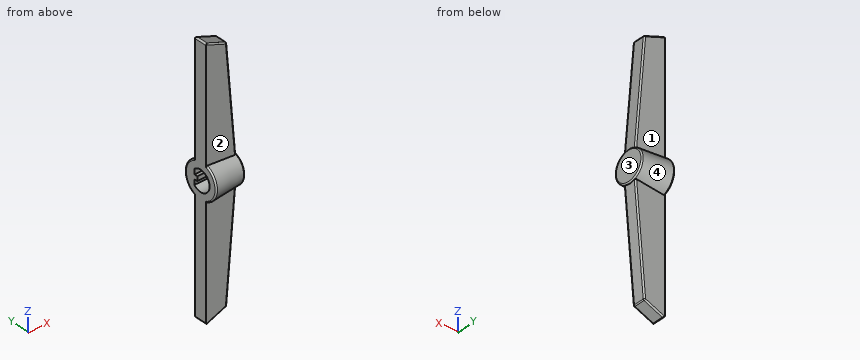
```python
from build123d import *

# Parameters (mm, degrees)
SKETCH028_R             = 6
SKETCH027_R             = 7
PAD010_DEPTH            = 2.5
FILLET002_R             = 0.5
FILLET003_R             = 0.5
FILLET004_R             = 0.5
POCKET009_DEPTH         = 8
BODY005_ROLL_ANGLE      = 90
BODY005_PLACEMENT_ANGLE = 90


with BuildPart() as part:
    # Sketch028 → AdditiveLoft section 0
    with BuildSketch(Plane.XY.offset(12)):
        Circle(SKETCH028_R)
    # Sketch027 → AdditiveLoft section 1
    with BuildSketch(Plane.XY):
        Circle(SKETCH027_R)
    loft()

    # Sketch029 → Pad010 (new body, symmetric)
    with BuildSketch(Plane.YZ):
        Polygon((0, 12), (46.829478, 8), (50, 0), (0, 0), (-50, 0), (-46.829478, 8), align=None)
    extrude(amount=PAD010_DEPTH, both=True)

    # Fillet002
    fillet002_edges = [part.edges().sort_by_distance(p)[0] for p in [
        (-6, 0, 12),
    ]]
    fillet(fillet002_edges, radius=FILLET002_R)

    # Fillet003
    fillet003_edges = [part.edges().sort_by_distance(p)[0] for p in [
        (-7, 0, 0),
        (5.766281, 3.968627, 0),
        (5.766281, -3.968627, 0),
    ]]
    fillet(fillet003_edges, radius=FILLET003_R)

    # Fillet004
    fillet004_edges = [part.edges().sort_by_distance(p)[0] for p in [
        (2.5, 26.163425, 9.765217),
        (-2.5, 26.163425, 9.765217),
        (-2.5, -26.163425, 9.765217),
        (2.5, -26.163425, 9.765217),
        (0, -46.829478, 8),
        (0, -50, 0),
        (-2.5, -48.414739, 4),
        (2.5, -48.414739, 4),
        (2.5, 48.414739, 4),
        (0, 46.829478, 8),
        (-2.5, 48.414739, 4),
        (0, 50, 0),
    ]]
    fillet(fillet004_edges, radius=FILLET004_R)

    # Sketch030 → Pocket009 (cut)
    with BuildSketch(Plane.XY):
        with BuildLine():
            Line((2.8, 2.856571), (2.8, 0.85))
            Line((2.8, 0.85), (1.5, 0.85))
            Line((1.5, 0.85), (1.5, -0.85))
            Line((1.5, -0.85), (2.8, -0.85))
            Line((2.8, -0.85), (2.8, -2.856571))
            ThreePointArc((2.8, 2.856571), (-4, 0), (2.8, -2.856571))
        make_face()
    extrude(amount=POCKET009_DEPTH, mode=Mode.SUBTRACT)


with BuildPart() as part_1:
    # Body005 roll: moved
    add(part.part.rotate(Axis((0, 0, 0), (1, 0, 0)), BODY005_ROLL_ANGLE))


with BuildPart() as part_2:
    # Body005 placement: moved
    add(part_1.part.moved(Location((53.5, 0, 0))).rotate(Axis((53.5, 0, 0), (0, 0, 1)), BODY005_PLACEMENT_ANGLE))


solid = part_2.part
```
Check sheet for the modelled part. Datum: model origin and axes. Units: mm. Face numbers are marked on the shaded views. Round coordinates to 2 decimals unless told otherwise and drop trailing zeros. Order: outer loops, then holes, each group sorted by start corner. A loop starts at its lowest first (then second) coordinate and runs counter-clockwise, first axis right, second up. Notation, with made-up numbers: (27, 63.25) -> (75, 63.25) arc R27 cw to (75, 95.25) -> close; hole circle Ø1 at (34, 15). An arc over 180 degrees is marked (long way). One line per item, written item: value. Start each with the question number.
Q1. Mould release check, pull along Y, two halves, no side actions. Record for the marked faces 1, 2, 3 and 4: pulls with the +Y half, pulls with the -Y half, needs draft (parallel to the pull), parting line crosses it, or undercut.
Q2. Cross-section at A-A (y = 0). Record the boundary of the cut face in (x, z), and give its area (3 significant figures).
Q3. Gauge pin test, flat ends, axial feed: pin 1 Ø5.5 at (x, z) = (61, -22) entering from -Y; pin 2 Ø1.4 at (x, y) = (58.5, 2) entering from -Z; pin 3 Ø1 at (x, y) = (59.5, 2) entering from +Z; pin 4 Ø7.5 at (y, z) = (-1.5, 0) entering from -X. Record the tip position at first contact, or that the pin passes through.
Q4. Thickness scan on line 1 (Z direction, x = 57.5, y = 0); line 2 (Z direction, x = 57.25, y = 0); line 3 (Y direction, x = 56.75, z = -45). Record the ranges inside material, lowest first.
Completed:
1. face 1: pulls with the +Y half
1. face 2: pulls with the -Y half
1. face 3: needs draft
1. face 4: parting line crosses it
2. outline: (53.5, -49.26) arc R0.5 ccw to (54.18, -49.73) -> (61.21, -46.94) arc R0.5 ccw to (61.53, -46.52) -> (64.98, -6.04) -> (65.04, -6.04) arc R0.5 ccw to (65.5, -5.54) -> (65.5, 5.54) arc R0.5 ccw to (65.04, 6.04) -> (64.98, 6.04) -> (61.53, 46.52) arc R0.5 ccw to (61.21, 46.94) -> (54.18, 49.73) arc R0.5 ccw to (53.5, 49.26) -> (53.5, 4) -> (61.5, 4) -> (61.5, -4) -> (53.5, -4) -> close
2. area: 901 mm²
3. pin 1: stops at y = -2.5
3. pin 2: stops at z = -48.3
3. pin 3: stops at z = 47.82
3. pin 4: stops at x = 53.5
4. line 1: z = -48.41 to -4, 4 to 48.41
4. line 2: z = -48.51 to -4, 4 to 48.51
4. line 3: y = -2.5 to 2.5
